Input: part model. Units: mm. Frame: model coordinates. A direction names the side the tool comes from. Give positions to 0.01 mm unless a question says otherwise; leave off trailing zeros. Loops run counter-clockwise (first coordinate to the right, second up) from the corner with the lowest first, then second, coordinate; pieces in that order, holes last. Notation, with made-up numbers: M 20.5,56.25 L 64.5,56.25 A18 cw 64.5,76.25 Z; hole C -10,36.5 d3. An arc over 180 degrees is marked long. Return JSON: item names as keys, results as strings. Group by question number.
```python
from build123d import *

# Parameters (mm, degrees)
EXTRUDE_1_DEPTH     = 10
SKETCH_2_R          = 8
EXTRUDE_2_DEPTH     = 40
SKETCH_5_R          = 15
EXTRUDE_4_DEPTH     = 10
EXTRUDE_3_DEPTH     = 30
CUT_EXTRUDE_1_REACH = 23.002
SKETCH_4_R          = 8


with BuildPart() as part:
    # Эскиз1 → Бобышка-Вытянуть1 (new body)
    with BuildSketch(Plane(origin=(0, 0, 0), x_dir=(0, 0, -1), z_dir=(1, 0, 0))):
        Polygon((0, 11.547005384), (-10, 5.773502692), (-10, -5.773502692), (0, -11.547005384), (10, -5.773502692), (10, 5.773502692), align=None)
    extrude(amount=EXTRUDE_1_DEPTH)

    # Эскиз2 → Бобышка-Вытянуть2 (add)
    with BuildSketch(Plane(origin=(10, 0, 0), x_dir=(0, 0, -1), z_dir=(1, 0, 0))):
        Circle(SKETCH_2_R)
    extrude(amount=EXTRUDE_2_DEPTH)

    # Эскиз5 → Бобышка-Вытянуть4 (add)
    with BuildSketch(Plane.ZY):
        Circle(SKETCH_5_R)
    extrude(amount=EXTRUDE_4_DEPTH)

    # Эскиз3 → Бобышка-Вытянуть3 (add)
    with BuildSketch(Plane.ZY.offset(10)):
        Polygon((0, 11.547005384), (-6.001748602, 8.081894213), (-6.001748602, -8.081894213), (0, -11.547005384), (5.991634546, -8.087733566), (5.991634546, 8.087733566), align=None)
    extrude(amount=EXTRUDE_3_DEPTH)

    # Эскиз4 → Вырез-Вытянуть1 (cut, up to next)
    with BuildSketch(Plane(origin=(0, 0, -6.001748602), x_dir=(-1, 0, 0), z_dir=(0, 0, -1)), mode=Mode.PRIVATE) as cut_extrude_1_sk1:
        with Locations((25, 0)):
            Circle(SKETCH_4_R)
    cut_extrude_1_tool1 = extrude(cut_extrude_1_sk1.sketch, amount=-CUT_EXTRUDE_1_REACH, mode=Mode.PRIVATE) & part.part
    add(cut_extrude_1_tool1.solids().sort_by_distance((-25, 0, -6.001749))[0], mode=Mode.SUBTRACT)


solid = part.part
```
Item 1: Section B-B, the plane z = -1.25. Return loops of the section in (x, y), then the cut area to 3 significant figures.
Item 2: Material intervals for line 1 (X direction, y = 13.5, z = -1); line 2 (X direction, y = -9.5, z = -1); line 3 (Z direction, x = -12, y = 2), sorted ascending. Write a range as from..to.
Item 3: Reachability of faces 4 (the face through (4.93, 8.62, -5.07)), 5 (the face through (4.93, 8.7, 4.93)), 6 (the face through (-18, 6, -6.002)), 7 (the face through (4.93, -8.7, -4.93)) from +Z, -Z, +X, -X, +Y, -Y: full face, straight path, thin tool, end or side. Return the list, or none.
Item 4: Pull-direction query (X, two-part tool) for faces 1 (the face through (50, 0, 0)), 2 (the face through (-24.79, -9.842, 2.954)), 3 (the face through (-18.651, -4.868, -0.089)); classes: pulls with the +X half, pulls with the -X half, needs draft (parallel to the pull), parting line crosses it, or undercut.
Item 5: Section A-A, the plane x = -25. Return loops of the section in (y, z).
Item 6: Section C-C, the plane x = -11.5. Return loops of the section in (y, z), then the cut area to 3 significant figures.
Item 7: First-contact query: pin 1 Ø8 at (x, z) = (23.5, -11) entering from +Y; pin 2 Ø5 at (x, y) = (33.5, -3.5) entering from +Z; pin 3 Ø8 at (x, y) = (6.5, -2.5) entering from -Z. Flat tips, straight axial feed; report the tip coordinate or a pass-through.
Item 8: Section D-D, the plane z = 7. Return loops of the section in (x, y), then the cut area to 3 significant figures.
Answer below:
{
 "1": {"outline": "M -40,-10.83 L -10,-10.83 L -10,-14.95 L 0,-14.95 L 0,-10.83 L 10,-10.83 L 10,-7.9 L 50,-7.9 L 50,7.9 L 10,7.9 L 10,10.83 L 0,10.83 L 0,14.95 L -10,14.95 L -10,10.83 L -40,10.83 Z; hole C -25,0 d16", "area": "1,600 mm^2"},
 "2": {"line 1": "-10..0", "line 2": "-40..10", "line 3": "-6..5.99"},
 "3": {"face 4": "-Z, +X, +Y", "face 5": "+Z, +X, +Y", "face 6": "-Z, -X, +Y, -Y", "face 7": "-Z, +X, -Y"},
 "4": {"face 1": "pulls with the +X half", "face 2": "needs draft", "face 3": "undercut"},
 "5": {"outline": "M -11.55,0 L -8.08,-6 L -8,-6 L -8,5.99 L -8.09,5.99 Z; M 8,-6 L 8.08,-6 L 11.55,0 L 8.09,5.99 L 8,5.99 Z"},
 "6": {"outline": "M -11.55,0 L -8.08,-6 L 8.08,-6 L 11.55,0 L 8.09,5.99 L -8.09,5.99 Z", "area": "235 mm^2"},
 "7": {"pin 1": "y = 3.87", "pin 2": "z = 7.94", "pin 3": "z = -10"},
 "8": {"outline": "M -10,-13.27 L 0,-13.27 L 0,-7.51 L 10,-7.51 L 10,-3.87 L 50,-3.87 L 50,3.87 L 10,3.87 L 10,7.51 L 0,7.51 L 0,13.27 L -10,13.27 Z", "area": "725 mm^2"}
}
